from build123d import *
from OCP.BRepFilletAPI import BRepFilletAPI_MakeChamfer

# Parameters (mm, degrees)
SKETCH4_W                = 12.46
SKETCH4_H                = 17.25
BOSS_EXTRUDE3_DEPTH      = 6
BOSS_EXTRUDE6_DEPTH      = 7.3
BOSS_EXTRUDE6_DEPTH_BACK = 17.25
SKETCH8_R                = 12.546781182
SKETCH8_R_2              = 11.15
BOSS_EXTRUDE4_DEPTH      = 17.25
SKETCH6_R                = 2
CUT_EXTRUDE1_DEPTH       = 5
CHAMFER1_SIZE            = 0.5
CHAMFER1_SIZE_2          = 0.866025404
SKETCH10_W               = 12.46
SKETCH10_H               = 23.7
CUT_EXTRUDE3_DEPTH       = 17.25
CUT_EXTRUDE4_REACH       = 43.938
SKETCH11_W               = 5
SKETCH11_H               = 3
BOSS_EXTRUDE7_START      = -7.3
BOSS_EXTRUDE7_DEPTH      = 7.3
BOSS_EXTRUDE9_START      = 10
BOSS_EXTRUDE9_DEPTH      = 10
BOSS_EXTRUDE10_DEPTH     = 25.093562364
SKETCH18_W               = 20
SKETCH18_H               = 12.438292938
CUT_EXTRUDE5_DEPTH       = 2
CUT_EXTRUDE6_DEPTH       = 57.41497434
CUT_EXTRUDE6_DEPTH_BACK  = 57.41497434
SKETCH19_R               = 1.25
FILLET1_R                = 10


with BuildPart() as part:
    # Sketch4 → Boss-Extrude3 (new body)
    with BuildSketch(Plane.XY):
        with Locations((0, -1.35)):
            Rectangle(SKETCH4_W, SKETCH4_H)
    extrude(amount=BOSS_EXTRUDE3_DEPTH)



with BuildPart() as body_2:
    # Sketch8 → Boss-Extrude6 (new, two sides: drawn at the far end of the back side and taken through both)
    with BuildSketch(Plane(origin=(0, -9.975, 0), x_dir=(-1, 0, 0), z_dir=(0, -1, 0)).offset(-BOSS_EXTRUDE6_DEPTH_BACK)):
        with Locations(Location((0, -23.55, 0), (0, 0, 90))):
            Circle(SKETCH8_R)
        with Locations(Location((0, -23.55, 0), (0, 0, 90))):
            Circle(SKETCH8_R_2, mode=Mode.SUBTRACT)
    extrude(amount=BOSS_EXTRUDE6_DEPTH + BOSS_EXTRUDE6_DEPTH_BACK)


with BuildPart() as part_1:
    add(part.part)

    add(body_2.part)  # Boss-Extrude4 merges body 2
    # Sketch5 → Boss-Extrude4 (add)
    with BuildSketch(Plane(origin=(0, 7.275, 0), x_dir=(1, 0, 0), z_dir=(0, 1, 0))):
        with BuildLine():
            Line((12.546781182, -23.55), (12.546781182, 0))
            Line((12.546781182, 0), (6.23, 0))
            Line((6.23, 0), (6.23, -29.7))
            Line((6.23, -29.7), (-6.23, -29.7))
            Line((-6.23, -29.7), (-6.23, 0))
            Line((-6.23, 0), (-12.546781182, 0))
            Line((-12.546781182, 0), (-12.546781182, -23.55))
            ThreePointArc((-12.546781182, -23.55), (0, -36.096781182), (12.546781182, -23.55))
        make_face()
    extrude(amount=-BOSS_EXTRUDE4_DEPTH)

    # Sketch6 → Cut-Extrude1 (cut)
    with BuildSketch(Plane(origin=(0, 7.275, 0), x_dir=(1, 0, 0), z_dir=(0, 1, 0))):
        with Locations(Location((0, -3.5, 0), (0, 0, 270))):
            Circle(SKETCH6_R)
        with Locations(Location((0, -32.2, 0), (0, 0, 270))):
            Circle(SKETCH6_R)
    extrude(amount=-CUT_EXTRUDE1_DEPTH, mode=Mode.SUBTRACT)

    # Chamfer1
    chamfer1_edges_1 = [part_1.edges().sort_by_distance(p)[0] for p in [
        (0, 7.275, 1.5),
    ]]
    chamfer1_side_1 = [part_1.faces().sort_by_distance(p)[0] for p in [
        (0, 7.275, 1.49),
    ]]
    chamfer1_edges_2 = [part_1.edges().sort_by_distance(p)[0] for p in [
        (0, 7.275, 30.2),
    ]]
    chamfer1_side_2 = [part_1.faces().sort_by_distance(p)[0] for p in [
        (0, 7.275, 30.19),
    ]]
    chamfer1 = BRepFilletAPI_MakeChamfer(part_1.part.solid().wrapped)
    for e in chamfer1_edges_1:
        chamfer1.Add(CHAMFER1_SIZE - 0.0001, CHAMFER1_SIZE_2 - 0.0001, e.wrapped, chamfer1_side_1[0].wrapped)
    for e in chamfer1_edges_2:
        chamfer1.Add(CHAMFER1_SIZE - 0.0001, CHAMFER1_SIZE_2 - 0.0001, e.wrapped, chamfer1_side_2[0].wrapped)
    add(Compound.cast(chamfer1.Shape()), mode=Mode.REPLACE)  # a hair under: the kernel refuses the full size

    # Sketch10 → Cut-Extrude3 (cut)
    with BuildSketch(Plane(origin=(0, 7.275, 0), x_dir=(1, 0, 0), z_dir=(0, 1, 0))):
        with Locations((0, -17.85)):
            Rectangle(SKETCH10_W, SKETCH10_H)
    extrude(amount=-CUT_EXTRUDE3_DEPTH, mode=Mode.SUBTRACT)

    # Sketch11 → Cut-Extrude4 (cut, up to next)
    with BuildSketch(Plane.XY.offset(36.096781182), mode=Mode.PRIVATE) as cut_extrude4_sk1:
        with Locations((0, -8.475)):
            Rectangle(SKETCH11_W, SKETCH11_H)
    cut_extrude4_tool1 = extrude(cut_extrude4_sk1.sketch, amount=-CUT_EXTRUDE4_REACH, mode=Mode.PRIVATE) & part_1.part
    add(cut_extrude4_tool1.solids().sort_by_distance((0, -8.475, 36.096781))[0], mode=Mode.SUBTRACT)

    # Sketch13 → Boss-Extrude7 (add)
    with BuildSketch(Plane.XZ.offset(17.275).offset(BOSS_EXTRUDE7_START)):
        with BuildLine():
            Line((-12.546781182, 23.55), (-12.546781182, 0))
            Line((-12.546781182, 0), (12.546781182, 0))
            Line((12.546781182, 0), (12.546781182, 23.55))
            ThreePointArc((12.546781182, 23.55), (0, 11.003218818), (-12.546781182, 23.55))
        make_face()
    extrude(amount=BOSS_EXTRUDE7_DEPTH)

    # Sketch15 → Boss-Extrude9 (add)
    with BuildSketch(Plane(origin=(0, 7.275, 0), x_dir=(1, 0, 0), z_dir=(0, 1, 0)).offset(BOSS_EXTRUDE9_START)):
        with BuildLine():
            Line((-12.546781182, 0), (12.546781182, 0))
            Line((12.546781182, 0), (12.546781182, -23.55))
            ThreePointArc((12.546781182, -23.55), (0, -36.096781182), (-12.546781182, -23.55))
            Line((-12.546781182, -23.55), (-12.546781182, 0))
        make_face()
        with BuildLine():
            Line((-6.23, -0.8), (6.23, -0.8))
            Line((6.23, -0.8), (6.23, -33.5))
            ThreePointArc((6.23, -33.5), (5.937106781, -34.207106781), (5.23, -34.5))
            Line((5.23, -34.5), (-5.23, -34.5))
            ThreePointArc((-5.23, -34.5), (-5.937106781, -34.207106781), (-6.23, -33.5))
            Line((-6.23, -33.5), (-6.23, -0.8))
        make_face(mode=Mode.SUBTRACT)
    extrude(amount=-BOSS_EXTRUDE9_DEPTH)

    # Sketch17 → Boss-Extrude10 (add)
    with BuildSketch(Plane(origin=(-12.546781182, 4.728218818, 0), x_dir=(0, -1, 0), z_dir=(1, 0, 0))):
        Polygon((26.478218818, 25), (26.478218818, 0), (-17.021781182, 0), (-17.021781182, 25), (-13.021781182, 25), (-13.021781182, 5), (22.478218818, 5), (22.478218818, 25), align=None)
    extrude(amount=BOSS_EXTRUDE10_DEPTH)

    # Sketch18 → Cut-Extrude5 (cut)
    with BuildSketch(Plane.ZX.offset(-17.75)):
        with Locations((-15, 0)):
            Rectangle(SKETCH18_W, SKETCH18_H)
    extrude(amount=-CUT_EXTRUDE5_DEPTH, mode=Mode.SUBTRACT)

    # Sketch19 → Cut-Extrude6 (cut, two sides: drawn at the far end of the back side and taken through both)
    with BuildSketch(Plane.ZX.offset(-19.75).offset(-CUT_EXTRUDE6_DEPTH_BACK)):
        with Locations((-20, 0)):
            Circle(SKETCH19_R)
    extrude(amount=CUT_EXTRUDE6_DEPTH + CUT_EXTRUDE6_DEPTH_BACK, mode=Mode.SUBTRACT)

    # Fillet1
    fillet1_edges = [part_1.edges().sort_by_distance(p)[0] for p in [
        (12.546781182, -19.75, -25),
        (-12.546781182, -19.75, -25),
        (12.546781182, 19.75, -25),
        (-12.546781182, 19.75, -25),
    ]]
    fillet(fillet1_edges, radius=FILLET1_R)


solid = part_1.part
Build history of the part. All positions in model axes, mm. A direction names the side the tool comes from. Round coordinates to 2 decimals unless told otherwise and drop trailing zeros. Loops run counter-clockwise (first coordinate to the right, second up) from the corner with the lowest first, then second, coordinate; pieces in that order, holes last. Notation, with made-up numbers: (6, 74) -> (13, 74) arc R27 cw to (13, 97) -> close; hole circle Ø1 at (10, -10). An arc over 180 degrees is marked (long way). One line per item, written item: value. Start each with the question number.
Q1. Cut at B-B on z = -12. List the corners of the cut face in (x, y), plus the area to 3 significant figures.
Q2. Cut at C-C on x = -4.5. List the corners of the cut face in (y, z) (3 decimals), plus the area to 3 significant figures.
Q3. 3-axis set-ups, long thin cutter, end or side, ignore diameter. For faces 4 (the face through (-8, 17.275, 14)), 5 (the face through (0.49, -13.57, 34.69)), 6 (the face through (0, -6.975, 33)), 7 (the face through (9, -17.75, -15)): which of +Z, -Z, +X, -X, +Y, -Y reach the whole face in a straight line?
Q4. Cut at D-D on z = -20. List the corners of the cut face in (x, y), plus the area to 3 significant figures.
Q5. Cut at A-A on y = 15. List the corners of the cut face in (x, z).
Q6. Two-plate mould, pull along Z, no slides. Class faces 1 (the face through (6.219, -19, -15)), 2 (the face through (0.276, 0.242, 36.094)), 3 (the face through (-0.479, -20.764, -18.845)): released by +Z, released by -Z, zero draft, split by the parting line, or undercut.
Q7. Drop flat-ended pins along their axis: pin 1 Ø2 at (x, y) = (-9, 6.5) entering from -Z; pin 2 Ø3 at (x, z) = (0.5, 4) entering from +Y; pin 3 Ø1.2 at (x, z) = (1, 32) entering from +Y (3 decimals). Give the stop position or say it passes through.
Q8. Probe line 1 along X through (y, z) = (5.15, 3.5); line 2 along Y through (x, z) = (-4.5, -11.5); line 3 along Y through (x, z) = (-10.5, -11). List the from-to ranges inside material, lowest first.
Computed:
1. outline: (-12.55, -21.75) -> (12.55, -21.75) -> (12.55, -17.75) -> (6.22, -17.75) -> (6.22, -19.75) -> (-6.22, -19.75) -> (-6.22, -17.75) -> (-12.55, -17.75) -> close; (-12.55, 17.75) -> (12.55, 17.75) -> (12.55, 21.75) -> (-12.55, 21.75) -> close
1. area: 176 mm²
2. outline: (-21.75, -24.807) -> (-19.75, -24.807) -> (-19.75, -5) -> (17.75, -5) -> (17.75, -24.807) -> (21.75, -24.807) -> (21.75, 0) -> (17.275, 0) -> (17.275, 0.8) -> (7.275, 0.8) -> (7.275, 6) -> (-9.975, 6) -> (-9.975, 13.348) -> (-17.275, 13.348) -> (-17.275, 0) -> (-21.75, 0) -> close; (-17.275, 33.752) -> (-9.975, 33.752) -> (-9.975, 29.7) -> (7.275, 29.7) -> (7.275, 34.5) -> (17.275, 34.5) -> (17.275, 35.262) -> (-17.275, 35.262) -> close
2. area: 660 mm²
3. face 4: +Z, +X, -X, +Y
3. face 5: -Y
3. face 6: +Z
3. face 7: -Z, +X, -X
4. outline: (-11.21, -21.75) -> (-1.25, -21.75) -> (-1.25, -19.75) -> (-6.22, -19.75) -> (-6.22, -17.75) -> (-11.21, -17.75) -> close; (-11.21, 17.75) -> (-1.25, 17.75) -> (-1.25, 21.75) -> (-11.21, 21.75) -> close; (1.25, -21.75) -> (11.21, -21.75) -> (11.21, -17.75) -> (6.22, -17.75) -> (6.22, -19.75) -> (1.25, -19.75) -> close; (1.25, 17.75) -> (11.21, 17.75) -> (11.21, 21.75) -> (1.25, 21.75) -> close
4. area: 139 mm²
5. outline: (-12.55, -5) -> (12.55, -5) -> (12.55, 23.55) arc R12.55 ccw to (-12.55, 23.55) -> close; hole (-6.23, 0.8) -> (6.23, 0.8) -> (6.23, 33.5) arc R1 ccw to (5.23, 34.5) -> (-5.23, 34.5) arc R1 ccw to (-6.23, 33.5) -> close
6. face 1: zero draft
6. face 2: released by +Z
6. face 3: undercut
7. pin 1: z = -5
7. pin 2: y = 6.77
7. pin 3: y = 2.275
8. line 1: -12.55 to -2, 2 to 12.55
8. line 2: -21.75 to -19.75, 17.75 to 21.75
8. line 3: -21.75 to -17.75, 17.75 to 21.75
